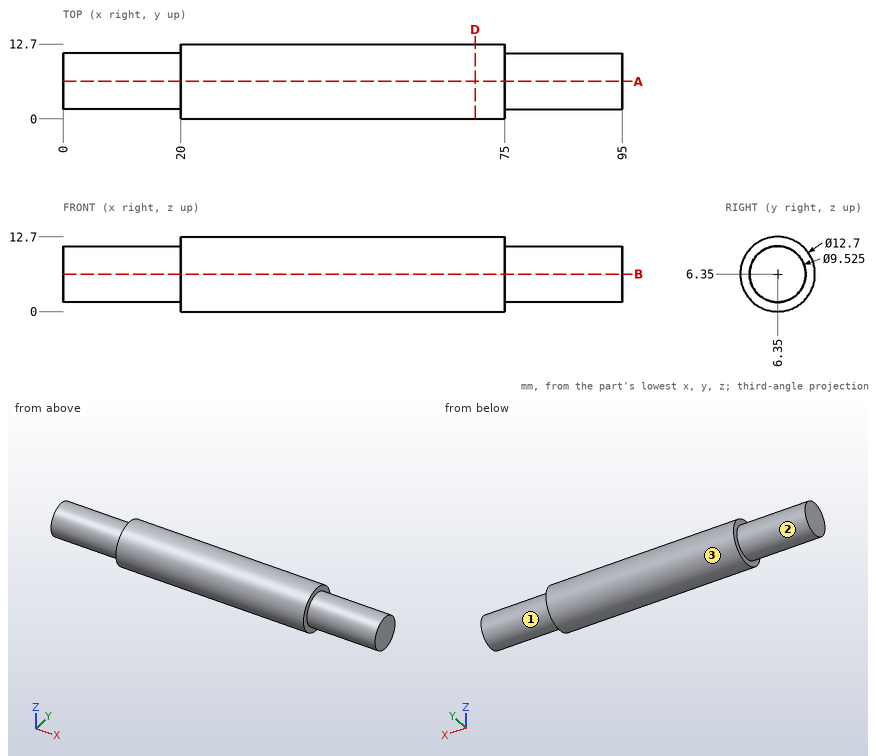
Print and shaded views of the part. All mm, measured from the part's lowest x, y and z. A direction names the side the tool comes from. Give positions to 0.01 mm unless a question says otherwise; leave off trailing zeros. Loops run counter-clockwise (first coordinate to the right, second up) from the corner with the lowest first, then second, coordinate; pieces in that order, holes last. Notation, with made-up numbers: (20.25, 16.5) - (38.25, 16.5) arc R13 cw to (38.25, 31.5) - close; hole circle Ø11 at (35.25, 60). An arc over 180 degrees is marked (long way). Use a Markdown table: item, result.
(1) Wall check: line 1 along Y through (x, z) = (16, 6.5); line 2 along X through (y, z) = (4.5, 11.75); line 3 along Z through (x, y) = (86, 6). Give the ranges that are in metal, low to high.
Taken from the geometry:
| item | result |
|---|---|
| line 1 | 1.59 to 11.11 |
| line 2 | 20 to 75 |
| line 3 | 1.6 to 11.1 |
(2) Band-saw the part on A-A (y = 6.35). Give the cut face in (x, z), and give its area (3 significant figures).
Taken from the geometry:
| item | result |
|---|---|
| outline | (0, 1.59) - (20, 1.59) - (20, 0) - (75, 0) - (75, 1.59) - (95, 1.59) - (95, 11.11) - (75, 11.11) - (75, 12.7) - (20, 12.7) - (20, 11.11) - (0, 11.11) - close |
| area | 1,080 mm2 |
(3) Drop flat-ended pins along their axis: pin 1 Ø1 at (x, y) = (60.5, 8) entering from +Z (3 decimals); pin 2 Ø1 at (x, z) = (41.5, 10.5) entering from -Y; pin 3 Ø3 at (x, y) = (80.5, 4.5) entering from +Z. Give the stop position or say it passes through.
Taken from the geometry:
| item | result |
|---|---|
| pin 1 | z = 12.595 |
| pin 2 | y = 1.15 |
| pin 3 | z = 11.1 |
(4) Band-saw the part on D-D (x = 70). Give the cut face in (y, z).
Taken from the geometry:
| item | result |
|---|---|
| outline | circle Ø12.7 at (6.35, 6.35) |
(5) Which spindle directions (+Z, -Z, +X, -X, +Y, -Y) get a long thin tool onto all of the face, cutting with end or side? Do the marked faces 1, 2 and 3. Say none if no direction does.
Taken from the geometry:
| item | result |
|---|---|
| face 1 | +X |
| face 2 | -X |
| face 3 | +X, -X |
